from build123d import *

# Parameters (mm, degrees)
CYLINDER008_R           = 3
CYLINDER008_DEPTH       = 4
CYLINDER009_R           = 2
CYLINDER009_DEPTH       = 11.5
CYLINDER007_R           = 3
CYLINDER007_DEPTH       = 4
CYLINDER006_R           = 2
CYLINDER006_DEPTH       = 11.5
CYLINDER004_R           = 2
CYLINDER004_DEPTH       = 10
CYLINDER005_R           = 3
CYLINDER005_DEPTH       = 7
CYLINDER003_R           = 2
CYLINDER003_DEPTH       = 10
CYLINDER_R              = 3
CYLINDER_DEPTH          = 7
CYLINDER002_R           = 5
CYLINDER002_DEPTH       = 56.5
CYLINDER002_PITCH_ANGLE = 90
BOX011_W                = 42
BOX011_H                = 5
BOX011_DEPTH            = 5
BOX007_W                = 42
BOX007_H                = 48
BOX007_DEPTH            = 7.5
BOX008_W                = 42
BOX008_H                = 3
BOX008_DEPTH            = 15
BOX015_W                = 10
BOX015_H                = 10
BOX015_DEPTH            = 7
BOX014_W                = 10
BOX014_H                = 10
BOX014_DEPTH            = 7
BOX020_W                = 2.5
BOX020_H                = 7.5
BOX020_DEPTH            = 10
BOX020_ROLL_ANGLE       = 45
BOX005_W                = 2.5
BOX005_H                = 5
BOX005_DEPTH            = 10
BOX018_W                = 5
BOX018_H                = 5
BOX018_DEPTH            = 10
BOX019_W                = 58
BOX019_H                = 13
BOX019_DEPTH            = 10
CYLINDER021_W           = 5
CYLINDER021_H           = 3
CYLINDER021_ANGLE       = 180
CYLINDER019_W           = 5
CYLINDER019_H           = 3
CYLINDER019_ANGLE       = 180
CYLINDER017_W           = 2.5
CYLINDER017_H           = 54
CYLINDER017_ANGLE       = 180
CYLINDER016_W           = 5
CYLINDER016_H           = 56.5
CYLINDER016_ANGLE       = 180
BOX017_W                = 5
BOX017_H                = 3
BOX017_DEPTH            = 54
BOX016_W                = 10
BOX016_H                = 3
BOX016_DEPTH            = 56.5
CYLINDER020_W           = 5
CYLINDER020_H           = 3
CYLINDER020_ANGLE       = 180
CYLINDER018_W           = 5
CYLINDER018_H           = 3
CYLINDER018_ANGLE       = 180
CYLINDER014_W           = 2.5
CYLINDER014_H           = 54
CYLINDER014_ANGLE       = 180
CYLINDER015_W           = 5
CYLINDER015_H           = 56.5
CYLINDER015_ANGLE       = 180
FUSION007_PITCH_ANGLE   = 90
FILLET_R                = 1
CHAMFER003_SIZE         = 7.95


with BuildPart() as cylinder011:
    # Cylinder008 → Cylinder008 (new body)
    with BuildSketch(Plane.XY.offset(7.5)):
        Circle(CYLINDER008_R)
    extrude(amount=CYLINDER008_DEPTH)


with BuildPart() as bolt_hole4:
    # Cylinder009 → Cylinder009 (new body)
    with BuildSketch(Plane.XY):
        Circle(CYLINDER009_R)
    extrude(amount=CYLINDER009_DEPTH)

    # Fusion004: union Cylinder011
    add(cylinder011.part)


with BuildPart() as bolt_hole4_1:
    # Fusion004 placement: moved
    add(bolt_hole4.part.moved(Location((28, 45, -9))))


with BuildPart() as cylinder008:
    # Cylinder007 → Cylinder007 (new body)
    with BuildSketch(Plane.XY.offset(7.5)):
        Circle(CYLINDER007_R)
    extrude(amount=CYLINDER007_DEPTH)


with BuildPart() as bolt_hole3:
    # Cylinder006 → Cylinder006 (new body)
    with BuildSketch(Plane.XY):
        Circle(CYLINDER006_R)
    extrude(amount=CYLINDER006_DEPTH)

    # Fusion003: union Cylinder008
    add(cylinder008.part)


with BuildPart() as bolt_hole3_1:
    # Fusion003 placement: moved
    add(bolt_hole3.part.moved(Location((28, 12, -9))))


with BuildPart() as cylinder006:
    # Cylinder004 → Cylinder004 (new body)
    with BuildSketch(Plane.XY):
        Circle(CYLINDER004_R)
    extrude(amount=CYLINDER004_DEPTH)


with BuildPart() as bolt_hole2:
    # Cylinder005 → Cylinder005 (new body)
    with BuildSketch(Plane.XY):
        Circle(CYLINDER005_R)
    extrude(amount=CYLINDER005_DEPTH)

    # Fusion002: union Cylinder006
    add(cylinder006.part)


with BuildPart() as bolt_hole2_1:
    # Fusion002 placement: moved
    add(bolt_hole2.part.moved(Location((52.5, 27, -8))))


with BuildPart() as cylinder001:
    # Cylinder003 → Cylinder003 (new body)
    with BuildSketch(Plane.XY):
        Circle(CYLINDER003_R)
    extrude(amount=CYLINDER003_DEPTH)


with BuildPart() as bolt_hole1:
    # Cylinder → Cylinder (new body)
    with BuildSketch(Plane.XY):
        Circle(CYLINDER_R)
    extrude(amount=CYLINDER_DEPTH)

    # Fusion001: union Cylinder001
    add(cylinder001.part)


with BuildPart() as bolt_hole1_1:
    # Fusion001 placement: moved
    add(bolt_hole1.part.moved(Location((3.5, 27, -8))))


with BuildPart() as cable_tunnel_outer_shell:
    # Cylinder002 → Cylinder002 (new body)
    with BuildSketch(Plane.XY):
        Circle(CYLINDER002_R)
    extrude(amount=CYLINDER002_DEPTH)


with BuildPart() as cable_tunnel_outer_shell_1:
    # Cylinder002 pitch: moved
    add(cable_tunnel_outer_shell.part.rotate(Axis((0, 0, 0), (0, 1, 0)), CYLINDER002_PITCH_ANGLE))


with BuildPart() as cable_tunnel_outer_shell_2:
    # Cylinder002 placement: moved
    add(cable_tunnel_outer_shell_1.part)


with BuildPart() as fill_cut1:
    # Box011 → Box011 (new body)
    with BuildSketch(Plane(origin=(7, 0, -5), x_dir=(1, 0, 0), z_dir=(0, 0, 1))):
        with Locations((21, 2.5)):
            Rectangle(BOX011_W, BOX011_H)
    extrude(amount=BOX011_DEPTH)

    # Cut: cut cable-tunnel-outer-shell
    add(cable_tunnel_outer_shell_2.part, mode=Mode.SUBTRACT)


with BuildPart() as base_plate1:
    # Box007 → Box007 (new body)
    with BuildSketch(Plane(origin=(7, 4, -5), x_dir=(1, 0, 0), z_dir=(0, 0, 1))):
        with Locations((21, 24)):
            Rectangle(BOX007_W, BOX007_H)
    extrude(amount=BOX007_DEPTH)


with BuildPart() as nema17_support:
    # Box008 → Box008 (new body)
    with BuildSketch(Plane(origin=(7, 52, -5), x_dir=(1, 0, 0), z_dir=(0, 0, 1))):
        with Locations((21, 1.5)):
            Rectangle(BOX008_W, BOX008_H)
    extrude(amount=BOX008_DEPTH)


with BuildPart() as hold2:
    # Box015 → Box015 (new body)
    with BuildSketch(Plane(origin=(47, 22, -5), x_dir=(1, 0, 0), z_dir=(0, 0, 1))):
        with Locations((5, 5)):
            Rectangle(BOX015_W, BOX015_H)
    extrude(amount=BOX015_DEPTH)


with BuildPart() as hold1:
    # Box014 → Box014 (new body)
    with BuildSketch(Plane(origin=(-1, 22, -5), x_dir=(1, 0, 0), z_dir=(0, 0, 1))):
        with Locations((5, 5)):
            Rectangle(BOX014_W, BOX014_H)
    extrude(amount=BOX014_DEPTH)


with BuildPart() as cut_endstop_cable45:
    # Box020 → Box020 (new body)
    with BuildSketch(Plane.XY):
        with Locations((1.25, 3.75)):
            Rectangle(BOX020_W, BOX020_H)
    extrude(amount=BOX020_DEPTH)


with BuildPart() as cut_endstop_cable45_1:
    # Box020 roll: moved
    add(cut_endstop_cable45.part.rotate(Axis((0, 0, 0), (1, 0, 0)), BOX020_ROLL_ANGLE))


with BuildPart() as cut_endstop_cable45_2:
    # Box020 placement: moved
    add(cut_endstop_cable45_1.part.moved(Location((27, -8, -4.5))))


with BuildPart() as cut_endstop_cable:
    # Box005 → Box005 (new body)
    with BuildSketch(Plane(origin=(27, -8, -2.5), x_dir=(1, 0, 0), z_dir=(0, 0, 1))):
        with Locations((1.25, 2.5)):
            Rectangle(BOX005_W, BOX005_H)
    extrude(amount=BOX005_DEPTH)


with BuildPart() as cut_cable_drop:
    # Box018 → Box018 (new body)
    with BuildSketch(Plane(origin=(49, 0, -2.5), x_dir=(1, 0, 0), z_dir=(0, 0, 1))):
        with Locations((2.5, 2.5)):
            Rectangle(BOX018_W, BOX018_H)
    extrude(amount=BOX018_DEPTH)


with BuildPart() as cut_open:
    # Box019 → Box019 (new body)
    with BuildSketch(Plane(origin=(-1, -8, 2.45), x_dir=(1, 0, 0), z_dir=(0, 0, 1))):
        with Locations((29, 6.5)):
            Rectangle(BOX019_W, BOX019_H)
    extrude(amount=BOX019_DEPTH)


with BuildPart() as obj1:
    # Cylinder021 → Cylinder021 (revolve)
    with BuildSketch(Plane(origin=(0, 1, 3), x_dir=(-1, 0, 0), z_dir=(0, 1, 0))):
        with Locations((2.5, 1.5)):
            Rectangle(CYLINDER021_W, CYLINDER021_H)
    revolve(axis=Axis((0, 1, 3), (0, 0, 1)), revolution_arc=CYLINDER021_ANGLE)


with BuildPart() as obj2:
    # Cylinder019 → Cylinder019 (revolve)
    with BuildSketch(Plane(origin=(0, 0, 3), x_dir=(-1, 0, 0), z_dir=(0, 1, 0))):
        with Locations((2.5, 1.5)):
            Rectangle(CYLINDER019_W, CYLINDER019_H)
    revolve(axis=Axis((0, 0, 3), (0, 0, 1)), revolution_arc=CYLINDER019_ANGLE)

    # Cut014: cut obj1
    add(obj1.part, mode=Mode.SUBTRACT)


with BuildPart() as cable_tunnel_inner_upper:
    # Cylinder017 → Cylinder017 (revolve)
    with BuildSketch(Plane(origin=(0, 0, 0), x_dir=(-1, 0, 0), z_dir=(0, 1, 0))):
        with Locations((1.25, 27)):
            Rectangle(CYLINDER017_W, CYLINDER017_H)
    revolve(axis=Axis((0, 0, 0), (0, 0, 1)), revolution_arc=CYLINDER017_ANGLE)


with BuildPart() as cable_tunnel_upper:
    # Cylinder016 → Cylinder016 (revolve)
    with BuildSketch(Plane(origin=(0, 0, 0), x_dir=(-1, 0, 0), z_dir=(0, 1, 0))):
        with Locations((2.5, 28.25)):
            Rectangle(CYLINDER016_W, CYLINDER016_H)
    revolve(axis=Axis((0, 0, 0), (0, 0, 1)), revolution_arc=CYLINDER016_ANGLE)

    # Cut018: cut cable-tunnel-inner-upper
    add(cable_tunnel_inner_upper.part, mode=Mode.SUBTRACT)

    # Cut019: cut obj2
    add(obj2.part, mode=Mode.SUBTRACT)


with BuildPart() as cable_tunnel_upper_1:
    # Cut019 placement: moved
    add(cable_tunnel_upper.part.moved(Location((0, -3, 0))))


with BuildPart() as cable_tunnel_middle_inner:
    # Box017 → Box017 (new body)
    with BuildSketch(Plane(origin=(-2.5, -3, 0), x_dir=(1, 0, 0), z_dir=(0, 0, 1))):
        with Locations((2.5, 1.5)):
            Rectangle(BOX017_W, BOX017_H)
    extrude(amount=BOX017_DEPTH)


with BuildPart() as cable_tunnel_middle:
    # Box016 → Box016 (new body)
    with BuildSketch(Plane(origin=(-5, -3, 0), x_dir=(1, 0, 0), z_dir=(0, 0, 1))):
        with Locations((5, 1.5)):
            Rectangle(BOX016_W, BOX016_H)
    extrude(amount=BOX016_DEPTH)

    # Cut020: cut cable-tunnel-middle-inner
    add(cable_tunnel_middle_inner.part, mode=Mode.SUBTRACT)


with BuildPart() as obj3:
    # Cylinder020 → Cylinder020 (revolve)
    with BuildSketch(Plane(origin=(0, -1, 3), x_dir=(1, 0, 0), z_dir=(0, -1, 0))):
        with Locations((2.5, 1.5)):
            Rectangle(CYLINDER020_W, CYLINDER020_H)
    revolve(axis=Axis((0, -1, 3), (0, 0, 1)), revolution_arc=CYLINDER020_ANGLE)


with BuildPart() as obj4:
    # Cylinder018 → Cylinder018 (revolve)
    with BuildSketch(Plane(origin=(0, 0, 3), x_dir=(1, 0, 0), z_dir=(0, -1, 0))):
        with Locations((2.5, 1.5)):
            Rectangle(CYLINDER018_W, CYLINDER018_H)
    revolve(axis=Axis((0, 0, 3), (0, 0, 1)), revolution_arc=CYLINDER018_ANGLE)

    # Cut015: cut obj3
    add(obj3.part, mode=Mode.SUBTRACT)


with BuildPart() as cable_tunnel_inner_lower:
    # Cylinder014 → Cylinder014 (revolve)
    with BuildSketch(Plane.XZ):
        with Locations((1.25, 27)):
            Rectangle(CYLINDER014_W, CYLINDER014_H)
    revolve(axis=Axis((0, 0, 0), (0, 0, 1)), revolution_arc=CYLINDER014_ANGLE)


with BuildPart() as holder_with_cable_tunnel:
    # Cylinder015 → Cylinder015 (revolve)
    with BuildSketch(Plane.XZ):
        with Locations((2.5, 28.25)):
            Rectangle(CYLINDER015_W, CYLINDER015_H)
    revolve(axis=Axis((0, 0, 0), (0, 0, 1)), revolution_arc=CYLINDER015_ANGLE)

    # Cut016: cut cable-tunnel-inner-lower
    add(cable_tunnel_inner_lower.part, mode=Mode.SUBTRACT)

    # Cut017: cut obj4
    add(obj4.part, mode=Mode.SUBTRACT)

    # Fusion007: union cable-tunnel-upper, cable-tunnel-middle
    add(cable_tunnel_upper_1.part)
    add(cable_tunnel_middle.part)


with BuildPart() as holder_with_cable_tunnel_1:
    # Fusion007 pitch: moved
    add(holder_with_cable_tunnel.part.rotate(Axis((0, 0, 0), (0, 1, 0)), FUSION007_PITCH_ANGLE))


with BuildPart() as holder_with_cable_tunnel_2:
    # Fusion007 placement: moved
    add(holder_with_cable_tunnel_1.part)

    # Cut021: cut cut-open
    add(cut_open.part, mode=Mode.SUBTRACT)

    # Cut022: cut cut-cable-drop
    add(cut_cable_drop.part, mode=Mode.SUBTRACT)

    # Cut023: cut cut-endstop-cable
    add(cut_endstop_cable.part, mode=Mode.SUBTRACT)

    # Cut024: cut cut-endstop-cable45
    add(cut_endstop_cable45_2.part, mode=Mode.SUBTRACT)

    # Fillet
    fillet_edges = [holder_with_cable_tunnel_2.edges().sort_by_distance(p)[0] for p in [
        (0, -5.487469, -0.25),
        (0, -1.5, -2.5),
        (0, 2.487469, -0.25),
    ]]
    fillet(fillet_edges, radius=FILLET_R)

    # Fusion008: union fill-cut1, base-plate1, nema17-support, hold2, hold1
    add(fill_cut1.part)
    add(base_plate1.part)
    add(nema17_support.part)
    add(hold2.part)
    add(hold1.part)

    # Cut025: cut bolt-hole1
    add(bolt_hole1_1.part, mode=Mode.SUBTRACT)

    # Cut026: cut bolt-hole2
    add(bolt_hole2_1.part, mode=Mode.SUBTRACT)

    # Cut027: cut bolt-hole3
    add(bolt_hole3_1.part, mode=Mode.SUBTRACT)

    # Cut028: cut bolt-hole4
    add(bolt_hole4_1.part, mode=Mode.SUBTRACT)

    # Chamfer003
    chamfer003_edges = [holder_with_cable_tunnel_2.edges().sort_by_distance(p)[0] for p in [
        (7, 22, -1.5),
        (7, 32, -1.5),
        (49, 32, -1.5),
        (49, 22, -1.5),
    ]]
    chamfer(chamfer003_edges, length=CHAMFER003_SIZE)


solid = holder_with_cable_tunnel_2.part
The model under review builds one solid part; all positions refer to its coordinate system, in mm. A direction names the side the tool comes from. Round coordinates to 2 decimals unless told otherwise and drop trailing zeros. Loops run counter-clockwise (first coordinate to the right, second up) from the corner with the lowest first, then second, coordinate; pieces in that order, holes last. Notation, with made-up numbers: (81.25, 87) -> (129.25, 87) arc R26 ccw to (129.25, 105) -> close; hole circle Ø10 at (-23.5, -30). An arc over 180 degrees is marked (long way). Write item = value, one per line. Start each with the question number.
Item 1: Take a section at C-C on y = 45. Give the boundary of the cut face in (x, z).
Item 2: Mouldability with a two-part tool opening along Z and no side actions: class faces 1 (the cylindrical face through (14.18, -5.49, -0.2)), 2 (the cylindrical face through (25, 12, 0)), 3 (the flat face through (1, 27, -1)) as released by +Z, released by -Z, zero draft, split by the parting line, or undercut.
Item 3: Take a section at D-D on x = 14.5. Give the boundary of the cut face in (y, z).
Item 4: Take a section at A-A on y = 27. Give the boundary of the cut face in (x, z), plus the area to 3 significant figures.
Item 5: Insertion check: pin 1 (6.5 mm diameter, centred on x = 29, y = 12.5, fed in from +Z); pin 2 (3.5 mm diameter, centred on x = 52.5, y = 27, fed in from -Z); pin 3 (2.5 mm diameter, centred on y = -6.5, z = -1.5, fed in from +X); pin 4 (4 mm diameter, centred on x = 52, y = 31.5, fed in from +Z). Each pin has a flat end and moves straight along its axis. Give the tip position at first contact, or say it passes through.
Item 6: Take a section at B-B on x = 28. Give the boundary of the cut face in (y, z).
Item 7: To check wall thickness, follow L1, parallel to Y at x = 28, z = -0.3; L2, parallel to X at y = 4, z = 0.75; L3, parallel to X at y = 27, z = -4. State the ranges of each line that lie inside material, in increasing order.
Item 8: For faces 4 (the cylindrical face through (25.79, 47.03, 0.47)), 5 (the flat face through (50, 27, -1)), 6 (the flat face through (13, -5, 2.45)), 7 (the flat face through (29.5, -7, 0)), 8 (the cylindrical face through (4.52, 3.52, -2.14)), list the 3-axis set-ups (+Z, -Z, +X, -X, +Y, -Y) from which the entire face can be reached by the end or side of a thin tool; tool diameter is ignored.
Result:
q1.outline = (7, -5) -> (26, -5) -> (26, -1.5) -> (25, -1.5) -> (25, 2.5) -> (7, 2.5) -> close; (30, -5) -> (49, -5) -> (49, 2.5) -> (31, 2.5) -> (31, -1.5) -> (30, -1.5) -> close
q2.face_1 = undercut
q2.face_2 = zero draft
q2.face_3 = released by -Z
q3.outline = (-7.36, 2.45) arc R5 ccw to (-3, -5) -> (55, -5) -> (55, 10) -> (52, 10) -> (52, 2.5) -> (4, 2.5) -> (4, 2.45) -> (0.5, 2.45) arc R2.5 cw to (0, -2.5) -> (-3, -2.5) arc R2.5 cw to (-3.5, 2.45) -> close
q4.outline = (-1, -5) -> (0.5, -5) -> (0.5, -1) -> (1.5, -1) -> (1.5, 2) -> (-1, 2) -> close; (5.5, -1) -> (6.5, -1) -> (6.5, -5) -> (49.5, -5) -> (49.5, -1) -> (50.5, -1) -> (50.5, 2) -> (49, 2) -> (49, 2.5) -> (7, 2.5) -> (7, 2) -> (5.5, 2) -> close; (54.5, -1) -> (55.5, -1) -> (55.5, -5) -> (57, -5) -> (57, 2) -> (54.5, 2) -> close
q4.area = 355 mm²
q5.pin_1 = 2.5
q5.pin_2 = through
q5.pin_3 = 56.5
q5.pin_4 = 2
q6.outline = (-6.78, -3.28) arc R5 ccw to (-3, -5) -> (10, -5) -> (10, -1.5) -> (9, -1.5) -> (9, 2.5) -> (4, 2.5) -> (4, 2.45) -> (0.5, 2.45) arc R2.5 cw to (0, -2.5) -> (-6, -2.5) -> close; (14, -5) -> (43, -5) -> (43, -1.5) -> (42, -1.5) -> (42, 2.5) -> (15, 2.5) -> (15, -1.5) -> (14, -1.5) -> close; (47, -5) -> (55, -5) -> (55, 10) -> (52, 10) -> (52, 2.5) -> (48, 2.5) -> (48, -1.5) -> (47, -1.5) -> close
q7.L1 = 2.48 to 9, 15 to 42, 48 to 55
q7.L2 = 0 to 3, 6 to 49, 54 to 56.5
q7.L3 = -1 to 0.5, 6.5 to 49.5, 55.5 to 57
q8.face_4 = +Z
q8.face_5 = -Z
q8.face_6 = +Z, +X, -X, -Y
q8.face_7 = +Z, -Y
q8.face_8 = none
